```python
from build123d import *

# Parameters (mm, degrees)
SKETCH1_W           = 546.1
SKETCH1_H           = 279.4
BOSS_EXTRUDE1_DEPTH = 6.35
SKETCH2_W           = 31.75
SKETCH2_H           = 155.575
SKETCH2_W_2         = 6.35
SKETCH2_H_2         = 222.25
SKETCH2_W_3         = 63.5
SKETCH2_H_3         = 53.975
SKETCH2_W_4         = 495.3
SKETCH2_H_4         = 6.35
CUT_EXTRUDE1_DEPTH  = 307.975051918
EXTRUDE2_DEPTH      = 63.5
SKETCH4_R           = 38.1
BOSS_EXTRUDE2_DEPTH = 63.5
SKETCH5_W           = 76.2
SKETCH5_H           = 35.56
BOSS_EXTRUDE3_DEPTH = 6.35


with BuildPart() as part:
    # Sketch1 → Boss-Extrude1 (new, symmetric)
    with BuildSketch(Plane(origin=(0, 0, 0), x_dir=(1, 0, 0), z_dir=(0, 1, 0))):
        Rectangle(SKETCH1_W, SKETCH1_H)
    extrude(amount=BOSS_EXTRUDE1_DEPTH, both=True)

    # Sketch2 → Cut-Extrude1 (cut, through all)
    with BuildSketch(Plane(origin=(0, 6.35, 0), x_dir=(1, 0, 0), z_dir=(0, 1, 0))):
        with Locations((0, -61.9125)):
            Rectangle(SKETCH2_W, SKETCH2_H)
        with Locations((-269.875, -28.575)):
            Rectangle(SKETCH2_W_2, SKETCH2_H_2)
        with Locations((53.975, -63.5)):
            Rectangle(SKETCH2_W_3, SKETCH2_H_3)
        with Locations((0, 136.525)):
            Rectangle(SKETCH2_W_4, SKETCH2_H_4)
        with Locations((269.875, -28.575)):
            Rectangle(SKETCH2_W_2, SKETCH2_H_2)
    extrude(amount=-CUT_EXTRUDE1_DEPTH, mode=Mode.SUBTRACT)

    # Sketch3 → Extrude2 (add)
    with BuildSketch(Plane.XZ.offset(6.35)):
        Polygon((222.25, -116.992783244), (155.686970507, -22.86), (-155.686970507, -22.86), (-222.25, -116.992783244), (-275.22182791, -136.272951858), (-273.05, -142.24), (-218.211919626, -122.28057104), (-152.4, -29.21), (152.4, -29.21), (218.211919626, -122.28057104), (273.05, -142.24), (275.22182791, -136.272951858), align=None)
    extrude(amount=EXTRUDE2_DEPTH)

    # Sketch4 → Boss-Extrude2 (add)
    with BuildSketch(Plane(origin=(0, 6.35, 0), x_dir=(1, 0, 0), z_dir=(0, 1, 0))):
        with Locations(Location((222.25, -95.25, 0), (0, 0, 90))):
            Circle(SKETCH4_R)
        with Locations(Location((-222.25, -95.25, 0), (0, 0, 90))):
            Circle(SKETCH4_R)
    extrude(amount=BOSS_EXTRUDE2_DEPTH)

    # Sketch5 → Boss-Extrude3 (add)
    with BuildSketch(Plane(origin=(0, 0, -139.7), x_dir=(-1, 0, 0), z_dir=(0, 0, -1))):
        with Locations((-234.95, -11.43)):
            Rectangle(SKETCH5_W, SKETCH5_H)
        with Locations((234.95, -11.43)):
            Rectangle(SKETCH5_W, SKETCH5_H)
    extrude(amount=BOSS_EXTRUDE3_DEPTH)


solid = part.part
```
Geometry check sheet. Reference: the model listing, model coordinates, mm. A direction names the side the tool comes from. Round coordinates to 2 decimals unless told otherwise and drop trailing zeros. Order: outer loops, then holes, each group sorted by start corner. A loop starts at its lowest first (then second) coordinate and runs counter-clockwise, first axis right, second up. Notation, with made-up numbers: (78, 23.5) - (106, 23.5) arc R21 ccw to (106, 57.5) - close; hole circle Ø11 at (47, 1.5). An arc over 180 degrees is marked (long way). Use a Markdown table: item, result. Add a question column.
1) Section check C-C (x = -124). Record the cut outline in (y, z), then the cut area to 3 significant figures.
2) Thickness scan on line 1 along Z through (x, y) = (43, 2.5); line 2 along Z through (x, y) = (-131, -25.5); line 3 along Y through (x, z) = (165.5, -66). Record the ranges inside material, lowest first.
3) Set-up check for faces 1 (the flat face through (2, -38, -22.86)), 2 (the flat face through (54, 0, 90.488)), 3 (the cylindrical face through (256.05, 37.66, 77.67)), 4 (the flat face through (-143, 0, 139.7)): record each of +Z, -Z, +X, -X, +Y, -Y from which the full face is reachable in a straight line by a thin tool's end or side.
4) Section check A-A (x = 58.5). Record the cut outline in (y, z).
5) Gauge pin test, flat ends, axial feed: P1, Ø1.9, axis at x = -242.5, z = -142, coming from the -Y side; P2, Ø1.5, axis at y = 29.5, z = 101, coming from the -X side; P3, Ø1.7, axis at x = -274, z = -138, coming from the +Y side. Record the tip position at first contact, or that the pin passes through.
6) Section check B-B (y = -24). Record the cut outline in (x, z).
7) Mould release check, pull along X, two halves, no side actions. Record for faces 5 (the flat face through (140, 0, 139.7)), 6 (the flat face through (-188.503, -37.656, -69.267)), 7 (the flat face through (-231, -11, -139.7)), 8 (the flat face through (-2, -38, -29.21)): released by +X, released by -X, zero draft, split by the parting line, or undercut.
8) Section check D-D (y = 25.5). Record the cut outline in (x, z), then the cut area to 3 significant figures.
Established:
| question | item | result |
|---|---|---|
| 1 | outline | (-69.85, -29.21) - (-6.35, -29.21) - (-6.35, -133.35) - (6.35, -133.35) - (6.35, 139.7) - (-6.35, 139.7) - (-6.35, -22.86) - (-69.85, -22.86) - close |
| 1 | area | 3,870 mm2 |
| 2 | line 1 | -133.35 to 36.51, 90.49 to 139.7 |
| 2 | line 2 | -29.21 to -22.86 |
| 2 | line 3 | -6.35 to 6.35 |
| 3 | face 1 | +Z, +X, -X, -Y |
| 3 | face 2 | +Y, -Y |
| 3 | face 3 | +Y |
| 3 | face 4 | +Z, +X, -X, +Y, -Y |
| 4 | outline | (-69.85, -29.21) - (-6.35, -29.21) - (-6.35, -133.35) - (6.35, -133.35) - (6.35, 36.51) - (-6.35, 36.51) - (-6.35, -22.86) - (-69.85, -22.86) - close; (-6.35, 90.49) - (6.35, 90.49) - (6.35, 139.7) - (-6.35, 139.7) - close |
| 5 | P1 | y = -29.21 |
| 5 | P2 | x = -260.02 |
| 5 | P3 | y = -6.35 |
| 6 | outline | (-275.22, -136.27) - (-273.05, -142.24) - (-273.05, -146.05) - (-196.85, -146.05) - (-196.85, -139.7) - (-266.07, -139.7) - (-218.21, -122.28) - (-152.4, -29.21) - (152.4, -29.21) - (218.21, -122.28) - (266.07, -139.7) - (196.85, -139.7) - (196.85, -146.05) - (273.05, -146.05) - (273.05, -142.24) - (275.22, -136.27) - (222.25, -116.99) - (155.69, -22.86) - (-155.69, -22.86) - (-222.25, -116.99) - close |
| 7 | face 5 | zero draft |
| 7 | face 6 | released by -X |
| 7 | face 7 | undercut |
| 7 | face 8 | undercut |
| 8 | outline | circle Ø76.2 at (-222.25, 95.25); circle Ø76.2 at (222.25, 95.25) |
| 8 | area | 9,120 mm2 |
